```python
from build123d import *

# Parameters (mm, degrees)
F0_W     = 6.2
F0_H     = 2
F0_H_2   = 12.6
F0_H_3   = 1.8
F0_H_4   = 5.8
F1_DEPTH = 1
F2_DEPTH = 6
F3_R     = 3
F4_DEPTH = 0.5
F5_DEPTH = 2
F6_SIZE  = 1


with BuildPart() as f1:
    # F0 (on Top) → F1 (new body)
    with BuildSketch(Plane.XY):
        with Locations((0, 15.1)):
            Rectangle(F0_W, F0_H)
        with Locations((0, -11.1)):
            Rectangle(F0_W, F0_H)
        Rectangle(F0_W, F0_H_2)
        with Locations((0, -7.3)):
            Rectangle(F0_W, F0_H)
        with Locations((0, -9.2)):
            Rectangle(F0_W, F0_H_3)
        with Locations((0, 7.3)):
            Rectangle(F0_W, F0_H)
        with Locations((0, 11.2)):
            Rectangle(F0_W, F0_H_4)
    extrude(amount=-F1_DEPTH)

    # F0 (on Top) → F2 (join)
    with BuildSketch(Plane.XY):
        with Locations((0, 7.3)):
            Rectangle(F0_W, F0_H)
        with Locations((0, -7.3)):
            Rectangle(F0_W, F0_H)
        with Locations((0, -11.1)):
            Rectangle(F0_W, F0_H)
    extrude(amount=F2_DEPTH)

    # F3
    f3_edges = [f1.edges().sort_by_distance(p)[0] for p in [
        (-3.1, 7.3, 6),
        (-3.1, -7.3, 6),
        (-3.1, -11.1, 6),
        (3.1, 7.3, 6),
        (3.1, -7.3, 6),
        (3.1, -11.1, 6),
    ]]
    fillet(f3_edges, radius=F3_R)

    # F0 (on Top) → F4 (join)
    with BuildSketch(Plane.XY):
        with Locations((0, -9.2)):
            Rectangle(F0_W, F0_H_3)
    extrude(amount=F4_DEPTH)

    # F0 (on Top) → F5 (join)
    with BuildSketch(Plane.XY):
        with Locations((0, 15.1)):
            Rectangle(F0_W, F0_H)
    extrude(amount=F5_DEPTH)

    # F6
    f6_edges = [f1.edges().sort_by_distance(p)[0] for p in [
        (0, 16.1, 2),
    ]]
    chamfer(f6_edges, length=F6_SIZE)


solid = f1.part
```
Read the model definition and answer for the solid it produces. Units are mm, in the model's axes. A direction names the side the tool comes from. Give positions to 0.01 mm unless a question says otherwise; leave off trailing zeros. Order: outer loops, then holes, each group sorted by start corner. A loop starts at its lowest first (then second) coordinate and runs counter-clockwise, first axis right, second up.
(1) For a pull along Y with two mould halves and no side action, classify faces 4 (the flat face through (0, 16.1, 0)), 5 (the flat face through (3.1, 1.8, -0.4)), 6 (the flat face through (0, 11, 0)) as released by +Y, released by -Y, zero draft, split by the parting line, or undercut.
(2) Find section A-A (z = 0.75). Give the vertices of the cut face in (x, y).
(3) Straight lines are drawn through the part: L1, parallel to Y at x = 0, z = 4.75; L2, parallel to Z at x = -0.5, y = -2.5; L3, parallel to X at y = -6.5, z = 4.75. For each, find the intervals that lie inside material, in ascending order.
(4) Given pin 1 (0.8 mm diameter, centred on x = -1, y = 14.5, fed in from +Z); pin 2 (1 mm diameter, centred on x = 2, z = 4.5, fed in from +Y); pin 3 (3 mm diameter, centred on x = -2.5, y = -4.5, fed in from +Z), each flat-ended and moving along its own axis, determine where each tip first touches the part or whether it passes through.
(5) Find section D-D (y = -9). Give the vertices of the cut face in (x, z).
(6) For faces 1 (the flat face through (0, -8.3, 3)), 2 (the flat face through (0, 14.6, 2)), 3 (the cylindrical face through (2.24, -11.09, 5.1)), determine the directions among +Z, -Z, +X, -X, +Y, -Y from which every point of the face is accessible in a straight line to the end or side of a thin tool.
(7) Find section B-B (z = 3.75). Give the vertices of the cut face in (x, y).
(8) Find section C-C (x = 2.5). Give the vertices of the cut face in (y, z).
Result sheet:
1. face 4: released by +Y
1. face 5: zero draft
1. face 6: undercut
2. outline: (-3.1, -12.1) - (3.1, -12.1) - (3.1, -10.1) - (-3.1, -10.1) - close; (-3.1, -8.3) - (3.1, -8.3) - (3.1, -6.3) - (-3.1, -6.3) - close; (-3.1, 6.3) - (3.1, 6.3) - (3.1, 8.3) - (-3.1, 8.3) - close; (-3.1, 14.1) - (3.1, 14.1) - (3.1, 16.1) - (-3.1, 16.1) - close
3. L1: y = -12.1 to -10.1, -8.3 to -6.3, 6.3 to 8.3
3. L2: z = -1 to 0
3. L3: x = -2.54 to 2.54
4. pin 1: stops at z = 2
4. pin 2: stops at y = 8.3
4. pin 3: stops at z = 0
5. outline: (-3.1, -1) - (3.1, -1) - (3.1, 0.5) - (-3.1, 0.5) - close
6. face 1: +Z, +X, -X
6. face 2: +Z, +X, -X, +Y
6. face 3: +Z, +X, +Y, -Y
7. outline: (-3, -12.1) - (3, -12.1) - (3, -10.1) - (-3, -10.1) - close; (-3, -8.3) - (3, -8.3) - (3, -6.3) - (-3, -6.3) - close; (-3, 6.3) - (3, 6.3) - (3, 8.3) - (-3, 8.3) - close
8. outline: (-12.1, -1) - (16.1, -1) - (16.1, 1) - (15.1, 2) - (14.1, 2) - (14.1, 0) - (8.3, 0) - (8.3, 4.8) - (6.3, 4.8) - (6.3, 0) - (-6.3, 0) - (-6.3, 4.8) - (-8.3, 4.8) - (-8.3, 0.5) - (-10.1, 0.5) - (-10.1, 4.8) - (-12.1, 4.8) - close
